The model under review builds one solid part; all positions refer to its coordinate system, in mm. A direction names the side the tool comes from. Round coordinates to 2 decimals unless told otherwise and drop trailing zeros. Order: outer loops, then holes, each group sorted by start corner. A loop starts at its lowest first (then second) coordinate and runs counter-clockwise, first axis right, second up.
```python
from build123d import *

# Parameters (mm, degrees)
CYLINDER001_R     = 9.1
CYLINDER001_DEPTH = 20
BOX_W             = 33
BOX_H             = 4
BOX_DEPTH         = 30
FILLET_R          = 14
FILLET005_R       = 1
CHAMFER_SIZE      = 6
BOX003_W          = 10
BOX003_H          = 10
BOX003_DEPTH      = 3.6
FILLET004_R       = 1.6
BOX002_W          = 10
BOX002_H          = 10
BOX002_DEPTH      = 3.6
FILLET003_R       = 1.6
BOX001_W          = 4
BOX001_H          = 21.8
BOX001_DEPTH      = 26.4
FILLET001_R       = 4
FILLET002_R       = 1


with BuildPart() as cilindro001:
    # Cylinder001 → Cylinder001 (new body)
    with BuildSketch(Plane(origin=(611, 168, 72), x_dir=(1, 0, 0), z_dir=(0, 1, 0))):
        Circle(CYLINDER001_R)
    extrude(amount=CYLINDER001_DEPTH)


with BuildPart() as chamfer_body:
    # Box → Box (new body)
    with BuildSketch(Plane(origin=(597, 176, 57), x_dir=(1, 0, 0), z_dir=(0, 0, 1))):
        with Locations((16.5, 2)):
            Rectangle(BOX_W, BOX_H)
    extrude(amount=BOX_DEPTH)

    # Fillet
    fillet_edges = [chamfer_body.edges().sort_by_distance(p)[0] for p in [
        (597, 178, 87),
        (597, 178, 57),
    ]]
    fillet(fillet_edges, radius=FILLET_R)

    # Fillet005
    fillet005_edges = [chamfer_body.edges().sort_by_distance(p)[0] for p in [
        (630, 178, 57),
    ]]
    fillet(fillet005_edges, radius=FILLET005_R)

    # Chamfer
    chamfer_edges = [chamfer_body.edges().sort_by_distance(p)[0] for p in [
        (630, 178, 87),
    ]]
    chamfer(chamfer_edges, length=CHAMFER_SIZE)


with BuildPart() as fillet004:
    # Box003 → Box003 (new body)
    with BuildSketch(Plane(origin=(621, 184.9, 59.2), x_dir=(1, 0, 0), z_dir=(0, 0, 1))):
        with Locations((5, 5)):
            Rectangle(BOX003_W, BOX003_H)
    extrude(amount=BOX003_DEPTH)

    # Fillet004
    fillet004_edges = [fillet004.edges().sort_by_distance(p)[0] for p in [
        (626, 184.9, 59.2),
        (626, 184.9, 62.8),
        (626, 194.9, 59.2),
        (626, 194.9, 62.8),
    ]]
    fillet(fillet004_edges, radius=FILLET004_R)


with BuildPart() as fillet004_1:
    # Fillet004 placement: moved
    add(fillet004.part.moved(Location((0, 0, 18))))


with BuildPart() as fillet003:
    # Box002 → Box002 (new body)
    with BuildSketch(Plane(origin=(621, 184.9, 59.2), x_dir=(1, 0, 0), z_dir=(0, 0, 1))):
        with Locations((5, 5)):
            Rectangle(BOX002_W, BOX002_H)
    extrude(amount=BOX002_DEPTH)

    # Fillet003
    fillet003_edges = [fillet003.edges().sort_by_distance(p)[0] for p in [
        (626, 184.9, 59.2),
        (626, 184.9, 62.8),
        (626, 194.9, 59.2),
        (626, 194.9, 62.8),
    ]]
    fillet(fillet003_edges, radius=FILLET003_R)


with BuildPart() as cut002:
    # Box001 → Box001 (new body)
    with BuildSketch(Plane(origin=(626, 176, 57), x_dir=(1, 0, 0), z_dir=(0, 0, 1))):
        with Locations((2, 10.9)):
            Rectangle(BOX001_W, BOX001_H)
    extrude(amount=BOX001_DEPTH)

    # Fillet001
    fillet001_edges = [cut002.edges().sort_by_distance(p)[0] for p in [
        (628, 197.8, 57),
        (628, 197.8, 83.4),
    ]]
    fillet(fillet001_edges, radius=FILLET001_R)

    # Fillet002
    fillet002_edges = [cut002.edges().sort_by_distance(p)[0] for p in [
        (626, 184.9, 83.4),
        (626, 197.8, 70.2),
        (626, 184.9, 57),
        (630, 184.9, 83.4),
        (630, 197.8, 70.2),
        (630, 184.9, 57),
    ]]
    fillet(fillet002_edges, radius=FILLET002_R)

    # Cut: cut Fillet003
    add(fillet003.part, mode=Mode.SUBTRACT)

    # Cut001: cut Fillet004
    add(fillet004_1.part, mode=Mode.SUBTRACT)

    # Fusion: union Chamfer body
    add(chamfer_body.part)

    # Cut002: cut Cilindro001
    add(cilindro001.part, mode=Mode.SUBTRACT)


solid = cut002.part
```
(1) Consider section A-A (z = 72). Write out the cut boundary in (x, y), and give its area (3 significant figures).
Data:
outline: (597, 176) - (601.9, 176) - (601.9, 180) - (597, 180) - close; (620.1, 176) - (630, 176) - (630, 196.8) arc R1 ccw to (629, 197.8) - (627, 197.8) arc R1 ccw to (626, 196.8) - (626, 180) - (620.1, 180) - close
area: 130 mm2
(2) Consider section B-B (y = 189). Write out the cut boundary in (x, z), and give its area (3 significant figures).
Data:
outline: (626, 58) arc R1 ccw to (627, 57) - (629, 57) arc R1 ccw to (630, 58) - (630, 59.2) - (626, 59.2) - close; (626, 62.8) - (630, 62.8) - (630, 77.2) - (626, 77.2) - close; (626, 80.8) - (630, 80.8) - (630, 82.4) arc R1 ccw to (629, 83.4) - (627, 83.4) arc R1 ccw to (626, 82.4) - close
area: 75.9 mm2
(3) Consider section D-D (y = 182.5). Write out the cut boundary in (x, z).
Data:
outline: (626, 58) arc R1 ccw to (627, 57) - (629, 57) arc R1 ccw to (630, 58) - (630, 82.4) arc R1 ccw to (629, 83.4) - (627, 83.4) arc R1 ccw to (626, 82.4) - close
(4) Insertion check: pin 1 (10 mm diameter, centred on x = 600.5, z = 82.5, fed in from +Y); pin 2 (8 mm diameter, centred on x = 611, y = 181, fed in from +Z); pin 3 (4.5 mm diameter, centred on x = 628.5, y = 190.5, fed in from +Z); pin 4 (3 mm diameter, centred on y = 179.5, z = 80.5, fed in from -X). Each pin has a flat end and moves straight along its axis. Give the tip position at first contact, or say it passes through.
Data:
pin 1: stops at y = 180
pin 2: stops at z = 87
pin 3: stops at z = 83.4
pin 4: stops at x = 598.35
(5) Consider section C-C (x = 607). Write out the cut boundary in (y, z), and give its area (3 significant figures).
Data:
outline: (176, 57.58) - (180, 57.58) - (180, 63.83) - (176, 63.83) - close; (176, 80.17) - (180, 80.17) - (180, 86.42) - (176, 86.42) - close
area: 49.9 mm2
(6) To check wall thickness, follow probe 1 along Z at (x, y) = (611, 179); probe 2 along X at (y, z) = (180.5, 82.5); probe 3 along Y at (x, z) = (601, 66.5). State the ranges of each line that lie inside material, in increasing order.
Data:
probe 1: z = 57 to 62.9, 81.1 to 87
probe 2: x = 626.01 to 629.99
probe 3: y = 176 to 180
(7) For faces 4 (the cylindrical face through (628.03, 185.36, 77.68)), 5 (the cylindrical face through (626.285, 186.997, 83.099)), 6 (the flat face through (626, 188, 70)), list the 3-axis set-ups (+Z, -Z, +X, -X, +Y, -Y) from which the entire face can be reached by the end or side of a thin tool; tool diameter is ignored.
Data:
face 4: +X, -X
face 5: +Z, -X, +Y
face 6: +Z, -Z, -X, +Y
(8) Draft analysis for pull direction Y (two halves, no side actions). For faces 1 (the cylindrical face through (628.03, 194.44, 80.32)), 2 (the cylindrical face through (626.285, 197.499, 70.071)), 3 (the flat face through (628, 185, 83.4)), state which applies: pulls with the +Y half, pulls with the -Y half, needs draft (parallel to the pull), parting line crosses it, or undercut.
Data:
face 1: undercut
face 2: pulls with the +Y half
face 3: needs draft
